Can you work these out from the model? Positions are in its coordinate system, mm. Give positions to 0.01 mm unless a question says otherwise; leave off trailing zeros. Loops run counter-clockwise (first coordinate to the right, second up) from the corner with the lowest first, then second, coordinate; pieces in that order, holes last. Notation, with made-up numbers: (-7, 54) - (22, 54) arc R28 ccw to (22, 92) - close; hole circle Ø6 at (-30, 70.5). An arc over 180 degrees is marked (long way). Answer in a Markdown table with one row per item.
Autodesk Inventor part; units mm, degrees
ref_plane "Work Plane1" through (-8.3929, 0, 0) normal (0, -0.866, -0.5) x (1, 0, 0)
ref_plane "YZ Plane" through (0, 0, 0) normal (1, 0, 0) x (0, 1, 0)
ref_plane "XZ Plane" through (0, 0, 0) normal (0, 1, 0) x (-1, 0, 0)
sketch "Sketch1" plane through (0, 0, 0) normal (1, 0, 0) x (0, 1, 0)
  line L0 (-4.6188, 0) -> (-2.3094, 4)
  line L1 (-2.3094, 4) -> (2.3094, 4)
  line L2 (2.3094, 4) -> (4.6188, 0)
  line L3 (4.6188, 0) -> (2.3094, -4)
  line L4 (2.3094, -4) -> (-2.3094, -4)
  line L5 (-2.3094, -4) -> (-4.6188, 0)
  point P0 (0, 0)
  point P1 (0, 0)
  dimension "d0" = 9.2376
extrude "Body" add sketch "Sketch1" along normal blind 4.7
sketch "Sketch2" plane through (0, 0, 0) normal (0, 0, 1) x (1, 0, 0)
  line L0 (0, 2.3094) -> (0, 4.6188)
  line L1 (0, 4.6188) -> (4.7, 4.6188)
  line L2 (4.7, 2.3094) -> (4.7, 4.6188)
  line L3 (-0.94, 0) -> (5.64, 0)
  line L4 (0.2886, 4.6188) -> (0, 4)
  line L5 (4.4114, 4.6188) -> (4.7, 4)
  dimension "d3" = 25
  dimension "d4" = 25
  dimension "d5" = 8
  dimension "d6" = 8
revolve "Chamfer1" cut sketch "Sketch2" angle 360 about axis through (-10, 0, 0) along (1, 0, 0)
sketch "Sketch3" plane through (4.7, 0, 0) normal (1, 0, 0) x (0, 0, -1)
  arc A0 (-2, -3.4641) -> (2, -3.4641) centre (0, 0) ccw
hole "Thread" at (4.7, 0, 0) direction (-1, 0, 0) diameter 4.134 end through all
chamfer "Chamfer2" distance 0.433 angle 30 1 edges at (4.7, 0, 2.067) measured on face at (4.7, 3.336, -0.083)
chamfer "Chamfer3" distance 0.433 angle 30 1 edges at (0, 0, 2.067) measured on face at (0, 3.336, -0.083)
ref_plane "Work Plane1" through (-8.3929, 0, 0) normal (0, -0.866, -0.5) x (1, 0, 0)
equation "\"d0\" = 1.1547 * SW"
equation "\"d1\" = KOH"
equation "\"d3\" = ANG1"
equation "\"d4\" = ANG2"
equation "\"d5\" = SW0"
equation "\"d6\" = SW01"
equation "\"d8\" = -0.5 * GD1 + 0.5 * NND"
equation "\"d40\" = -0.5 * GD1 + 0.5 * NND"
equation "\"d10\" = -0.5 * GD1 + 0.5 * NND"
equation "\"d41\" = -0.5 * GD1 + 0.5 * NND"
equation "\"ANG1\" = 25deg"
equation "\"ANG2\" = 25deg"
equation "\"NND\" = 5"
equation "\"KOH\" = 4.7"
equation "\"SW\" = 8"
equation "\"SW0\" = SW"
equation "\"SW01\" = SW"
equation "\"GUL\" = 0.541266 * PTC"
equation "\"THREADDIA\" = 5"
equation "\"TOA\" = 30deg"
equation "\"PTC\" = 0.8"
equation "\"E0\" = 1.155 * SW"
equation "\"GAL\" = 0.541266 * PTC"
equation "\"SD2\" = 0"
equation "\"WFT\" = 0"
properties part number "ANSI B 18.2.4.1 M - M5 x 0.8" material "Steel, Mild"
Q1. Imagine slicing it at A-A, the plane x = 2.15. Write out the boundary of the cut face in (y, z).
Checked values:
| item | result |
|---|---|
| outline | (-4.62, 0) - (-2.31, -4) - (2.31, -4) - (4.62, 0) - (2.31, 4) - (-2.31, 4) - close; hole circle Ø4.13 at (0, 0) |
Q2. If I drill on line 1 (Z direction, x = 1.55, y = 0); line 2 (Z direction, x = 3.5, y = -0.5); line 3 (Y direction, x = 1.05, z = 0.75), over which ranges is the centre line in solid material (lowest first)? Write a range as [from, to].
Checked values:
| item | result |
|---|---|
| line 1 | z = [-4, -2.07], [2.07, 4] |
| line 2 | z = [-4, -2.01], [2.01, 4] |
| line 3 | y = [-4.19, -1.93], [1.93, 4.19] |
Q3. If we mould it in two halves opening along Y, with no side actions, what happens to faces 1 (the face through (2.32, 1.26, 1.64)), 2 (the face through (2.317, -3.448, -2.028)), 3 (the face through (2, 0, -4)), 4 (the face through (0.07, 2.08, 3.59))? For each: released by +Y, released by -Y, zero draft, split by the parting line, or undercut.
Checked values:
| item | result |
|---|---|
| face 1 | undercut |
| face 2 | released by -Y |
| face 3 | zero draft |
| face 4 | released by +Y |
